from build123d import *

# Parameters (mm, degrees)
REVOLUTION_ANGLE    = -180
BODY001_ROLL_ANGLE  = -180
BODY001_PITCH_ANGLE = -60


with BuildPart() as part:
    # Sketch → Revolution (revolve)
    with BuildSketch(Plane.XZ):
        with BuildLine():
            Line((43.30127, -25), (43.30127, -12.5))
            ThreePointArc((43.30127, 12.5), (30.80127, 0), (43.30127, -12.5))
            Line((43.30127, 12.5), (43.30127, 25))
            Line((43.30127, 25), (32.475953, 31.25))
            ThreePointArc((10.825318, 43.75), (15.400635, 26.674682), (32.475953, 31.25))
            Line((10.825318, 43.75), (0, 50))
            Line((0, 50), (0, -50))
            Line((0, -50), (10.825318, -43.75))
            ThreePointArc((32.475953, -31.25), (15.400635, -26.674682), (10.825318, -43.75))
            Line((32.475953, -31.25), (43.30127, -25))
        make_face()
    revolve(axis=Axis((0, 0, 0), (0, 0, 1)), revolution_arc=REVOLUTION_ANGLE)


with BuildPart() as part_1:
    # Body001 roll: moved
    add(part.part.rotate(Axis((0, 0, 0), (1, 0, 0)), BODY001_ROLL_ANGLE))


with BuildPart() as part_2:
    # Body001 pitch: moved
    add(part_1.part.rotate(Axis((0, 0, 0), (0, 1, 0)), BODY001_PITCH_ANGLE))


with BuildPart() as part_3:
    # Body001 placement: moved
    add(part_2.part)


solid = part_3.part
Verification items for the finished model (mm, model axes). Coordinates: 2 decimals unless noted, no trailing zeros.
Item 1: Section check A-A, the plane z = -29. Give the number of separate pieces and of enclosed holes in the cut face, then the cut area to 3 significant figures.
Filled in:
separate pieces: 3
enclosed holes: 0
area: 865 mm2
Item 2: Depth check by flat-ended pin: pin 1 (1.5 mm diameter, centred on x = 18.5, y = 37, fed in from -Z); pin 2 (8 mm diameter, centred on y = 36, z = -18.5, fed in from +X); pin 3 (1 mm diameter, centred on y = 27.5, z = -13, fed in from +X); pin 4 (5 mm diameter, centred on x = -21, z = -27, fed in from -Y). Enter the tip coordinate at first touch or a pass-through.
Filled in:
pin 1: stops at z = -24.48
pin 2: stops at x = 26.58
pin 3: stops at x = 23.48
pin 4: stops at y = 0
Item 3: Material ranges on L1, parallel to Z at x = -8, y = 19.5; L2, parallel to Y at x = -19, z = 10; L3, parallel to X at y = 32.5, z = -9, recorded low to high.
Filled in:
L1: z = -40.02 to -38.78, -24.75 to 42.27
L2: y = 0 to 43.29
L3: x = -35.39 to -17.24, 3.13 to 30.32
